Geometry: final body of the model. Coordinates: model frame, mm. A direction names the side the tool comes from. Give positions to 0.01 mm unless a question says otherwise; leave off trailing zeros. Write each loop counter-clockwise with the first axis right and the second up, starting at its lowest first coordinate (ties: lowest second). Pieces come first, ordered by that corner, then holes.
from build123d import *

# Parameters (mm, degrees)
F1_DEPTH = 10
F2_R     = 5
F3_DEPTH = 25
F5_DEPTH = 25
F6_R     = 1.5
F7_DEPTH = 25
F8_R     = 2.5
F9_DEPTH = 35


with BuildPart() as f1:
    # F0 (on Top) → F1 (new body)
    with BuildSketch(Plane.XY):
        with BuildLine():
            ThreePointArc((-6, 0), (0, -6), (6, 0))
            Line((6, 0), (-6, 0))
        make_face()
        with BuildLine():
            Line((-6, 0), (6, 0))
            ThreePointArc((6, 0), (0, 6), (-6, 0))
        make_face()
        with BuildLine():
            Line((6, -20), (6, 0))
            ThreePointArc((6, 0), (0, -6), (-6, 0))
            Line((-6, 0), (-6, -20))
            Line((-6, -20), (6, -20))
        make_face()
    extrude(amount=F1_DEPTH)

    # F2 (on face) → F3 (cut)
    with BuildSketch(Plane.XY.offset(10)):
        Circle(F2_R)
    extrude(amount=-F3_DEPTH, mode=Mode.SUBTRACT)

    # F4 (on face) → F5 (cut)
    with BuildSketch(Plane.XY.offset(10)):
        Polygon((-4, -7), (-4, -18), (4, -18), (4, -7), (0, -7), align=None)
    extrude(amount=-F5_DEPTH, mode=Mode.SUBTRACT)

    # F6 (on face) → F7 (cut)
    with BuildSketch(Plane.XZ.offset(7)):
        with Locations((0, 5)):
            Circle(F6_R)
    extrude(amount=-F7_DEPTH, mode=Mode.SUBTRACT)

    # F8 (on face) → F9 (join)
    with BuildSketch(Plane.XZ.offset(20)):
        with Locations((0, 5)):
            Circle(F8_R)
    extrude(amount=F9_DEPTH)


solid = f1.part
Q1. Section B-B on z = 1. Output: boundary loops of the cut face in (x, y), plus the area to 3 significant figures.
Filled sheet:
outline: (-6, -20) - (6, -20) - (6, 0) arc R6 ccw to (-6, 0) - close; hole circle Ø10 at (0, 0); hole (-4, -18) - (4, -18) - (4, -7) - (-4, -7) - close
area: 130 mm2
Q2. Access query for faces 4 (the flat face through (0, -18, 5)), 5 (the cylindrical face through (-0.33, -37.25, 7.48)), 6 (the flat face through (-0.1, -6.8, 0)), 7 (the cylindrical face through (1.43, 5.38, 5.45)). Directions: +Z, -Z, +X, -X, +Y, -Y. A direction counts if a zero-diameter tool reaches every point of the face in a straight line with its end or side. Return the directions, or none.
Filled sheet:
face 4: +Z, -Z
face 5: -Y
face 6: -Z, +X, -X, +Y, -Y
face 7: +Y
Q3. Pull-direction query (Z, two-part tool) for faces 1 (the cylindrical face through (-1.5, -5.9, 5.07)), 2 (the flat face through (-0.1, -6.8, 10)), 3 (the flat face through (0, -55, 5)); classes: released by +Z, released by -Z, zero draft, split by the parting line, or undercut.
Filled sheet:
face 1: undercut
face 2: released by +Z
face 3: zero draft
Q4. Section C-C on y = -24. Output: boundary loops of the cut face in (x, z), plus the area to 3 significant figures.
Filled sheet:
outline: circle Ø5 at (0, 5)
area: 19.6 mm2
Q5. Pin query (flat end, axial travel): P1, Ø1, axis at x = 4.5, z = 1.5, coming from the -Y side; P2, Ø3, axis at y = -37.5, z = 5, coming from the -X side; P3, Ø1.5, axis at x = -3, z = 1.5, coming from the +Y side; P4, Ø6, axis at x = 0, y = 0, coming from the -Z side. Return the tip coordinate at first contact, or that it passes through.
Filled sheet:
P1: stops at y = -20
P2: stops at x = -2.5
P3: stops at y = 5.56
P4: passes through
Q6. Ray query, line 1 along Y through (x, z) = (0.25, 1); line 2 along Y through (x, z) = (3.75, 6.25); line 3 along Z through (x, y) = (0, 5.4). Return the intervals inside material, ascending.
Filled sheet:
line 1: y = -20 to -18, -7 to -4.99, 4.99 to 5.99
line 2: y = -20 to -18, -7 to -3.31, 3.31 to 4.68
line 3: z = 0 to 3.5, 6.5 to 10
Q7. Section D-D on z = 5. Output: boundary loops of the cut face in (x, y).
Filled sheet:
outline: (-6, -20) - (-2.5, -20) - (-2.5, -55) - (2.5, -55) - (2.5, -20) - (6, -20) - (6, 0) arc R6 ccw to (1.5, 5.81) - (1.5, 4.77) arc R5 cw to (1.5, -4.77) - (1.5, -7) - (4, -7) - (4, -18) - (-4, -18) - (-4, -7) - (-1.5, -7) - (-1.5, -4.77) arc R5 cw to (-1.5, 4.77) - (-1.5, 5.81) arc R6 ccw to (-6, 0) - close
Q8. Section A-A on x = 0.75. Output: boundary loops of the cut face in (y, z).
Filled sheet:
outline: (-55, 2.62) - (-20, 2.62) - (-20, 0) - (-18, 0) - (-18, 10) - (-20, 10) - (-20, 7.38) - (-55, 7.38) - close; (-7, 0) - (-4.94, 0) - (-4.94, 3.7) - (-7, 3.7) - close; (-7, 6.3) - (-4.94, 6.3) - (-4.94, 10) - (-7, 10) - close; (4.94, 0) - (5.95, 0) - (5.95, 3.7) - (4.94, 3.7) - close; (4.94, 6.3) - (5.95, 6.3) - (5.95, 10) - (4.94, 10) - close
